Model file for the job. Use its own axes, mm. Face numbers are marked on the shaded views. Give positions to 0.01 mm unless a question says otherwise; leave off trailing zeros. Loops run counter-clockwise (first coordinate to the right, second up) from the corner with the lowest first, then second, coordinate; pieces in that order, holes last. Notation, with made-up numbers: M 41,56 L 71,56 A31 cw 71,90 Z; hole C 87.5,-5.5 d4. An arc over 180 degrees is marked long. Answer in a Markdown table with one row per item.
```python
from build123d import *

# Parameters (mm, degrees)
BOSS_EXTRUDE1_DEPTH = 5
BOSS_EXTRUDE2_DEPTH = 5


with BuildPart() as part:
    # Sketch1 → Boss-Extrude1 (new body)
    with BuildSketch(Plane.XY):
        Polygon((-10, 0), (10, 0), (20, -80), (-20, -80), align=None)
    extrude(amount=BOSS_EXTRUDE1_DEPTH)

    # Sketch2 → Boss-Extrude2 (add)
    with BuildSketch(Plane.XY):
        with BuildLine():
            Line((20, -80), (13.357757603, -26.862060826))
            ThreePointArc((13.357757603, -26.862060826), (0, -30), (-13.357757603, -26.862060826))
            Line((-13.357757603, -26.862060826), (-20, -80))
            Line((-20, -80), (20, -80))
        make_face()
    extrude(amount=-BOSS_EXTRUDE2_DEPTH)


solid = part.part
```
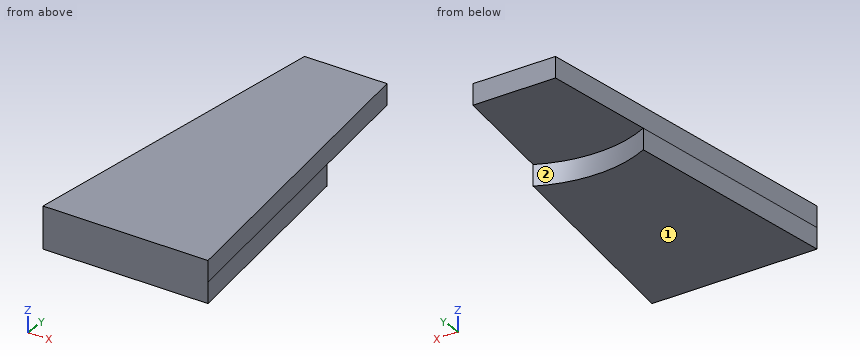
(1) Wall check: L1, parallel to Z at x = 2.5, y = -26; L2, parallel to X at y = -31, z = 3.5 (3 decimals); L3, parallel to Y at x = -9, z = -0.5. Give the ranges that are in metal, low to high.
Established:
| item | result |
|---|---|
| L1 | z = 0 to 5 |
| L2 | x = -13.875 to 13.875 |
| L3 | y = -80 to -28.62 |
(2) Saw through at B-B, the plane x = -15.5. Give the cut face in (y, z), and give its area (3 significant figures).
Established:
| item | result |
|---|---|
| outline | M -80,-5 L -44,-5 L -44,5 L -80,5 Z |
| area | 360 mm2 |
(3) Mould opens along X. For the marked faces 1 and 2 say: pulls with the +X half, pulls with the -X half, needs draft (parallel to the pull), parting line crosses it, or undercut.
Established:
| item | result |
|---|---|
| face 1 | needs draft |
| face 2 | undercut |
(4) Saw through at A-A, the plane y = -44. Give the cut face in (x, z).
Established:
| item | result |
|---|---|
| outline | M -15.5,-5 L 15.5,-5 L 15.5,5 L -15.5,5 Z |
(5) Saw through at C-C, the plane z = -2.25. Give the cut face in (x, y), and give its area (3 significant figures).
Established:
| item | result |
|---|---|
| outline | M -20,-80 L 20,-80 L 13.36,-26.86 A30 cw -13.36,-26.86 Z |
| area | 1,720 mm2 |
(6) Flat gauge pins, fed straight in: P1, Ø13.5, axis at x = 0.5, y = -11.5, coming from the -Z side; P2, Ø1, axis at y = -68.5, z = 0.5, coming from the -X side (3 decimals); P3, Ø1, axis at y = -39, z = -3, coming from the -X side. Where does each tip first touch, or does it go through?
Established:
| item | result |
|---|---|
| P1 | stops at z = 0 |
| P2 | stops at x = -18.625 |
| P3 | stops at x = -14.94 |
(7) Saw through at D-D, the plane y = -34. Give the cut face in (x, z).
Established:
| item | result |
|---|---|
| outline | M -14.25,-5 L 14.25,-5 L 14.25,5 L -14.25,5 Z |
